```python
from build123d import *

# Parameters (mm, degrees)
BOSS_EXTRU_1_DEPTH             = 15
ESQUISSE3_R                    = 4
BOSS_EXTRU_2_DEPTH             = 20
ESQUISSE4_R                    = 4
BOSS_EXTRU_3_DEPTH             = 20
TROU_TARAUD_M5X0_85_AT_2_COUNT = 2
TROU_TARAUD_M5X0_85_AT_2_PITCH = 44.72135955
ENL_V_START                    = -19
ESQUISSE13_R                   = 4
ESQUISSE13_R_2                 = 3
ENL_V_MAT_EXTRU_1_DEPTH        = 19


with BuildPart() as part:
    # Esquisse1 → Boss.-Extru.1 (new, symmetric)
    with BuildSketch(Plane.XY):
        Polygon((0, 60), (30, 60), (30, 30), (60, 30), (60, 0), (0, 0), align=None)
    extrude(amount=BOSS_EXTRU_1_DEPTH, both=True)

    # Esquisse3 → Boss.-Extru.2 (add)
    with BuildSketch(Plane(origin=(0, 60, 0), x_dir=(-1, 0, 0), z_dir=(0, 1, 0))):
        with Locations(Location((-15, 0, 0), (0, 0, 270))):
            Circle(ESQUISSE3_R)
    extrude(amount=BOSS_EXTRU_2_DEPTH)

    # Esquisse4 → Boss.-Extru.3 (add)
    with BuildSketch(Plane(origin=(60, 0, 0), x_dir=(0, 0, -1), z_dir=(1, 0, 0))):
        with Locations(Location((0, 15, 0), (0, 0, 180))):
            Circle(ESQUISSE4_R)
    extrude(amount=BOSS_EXTRU_3_DEPTH)

    # Esquisse8 → Trou taraudé M5x0.82 (revolve, cut)
    with BuildSketch(Plane(origin=(45, 5, 15), x_dir=(0, -1, 0), z_dir=(1, 0, 0))):
        Polygon((0, 0), (0, 8.2618073), (2.1, 7), (2.1, 0), align=None)
    trou_taraud_m5x0_82 = revolve(axis=Axis((45, 5, 21.35), (0, 0, -1)), mode=Mode.SUBTRACT)

    # Esquisse9 → Trou taraudé M5x0.83 (revolve, cut)
    with BuildSketch(Plane(origin=(45, 25, 15), x_dir=(0, -1, 0), z_dir=(1, 0, 0))):
        Polygon((0, 0), (0, 8.2618073), (2.1, 7), (2.1, 0), align=None)
    trou_taraud_m5x0_83 = revolve(axis=Axis((45, 25, 21.35), (0, 0, -1)), mode=Mode.SUBTRACT)

    # Esquisse10 → Trou taraudé M5x0.84 (revolve, cut)
    with BuildSketch(Plane(origin=(5, 45, 15), x_dir=(0, -1, 0), z_dir=(1, 0, 0))):
        Polygon((0, 0), (0, 8.2618073), (2.1, 7), (2.1, 0), align=None)
    trou_taraud_m5x0_84 = revolve(axis=Axis((5, 45, 21.35), (0, 0, -1)), mode=Mode.SUBTRACT)

    # Esquisse12 → Trou taraudé M5x0.85 (revolve, cut)
    with BuildSketch(Plane(origin=(25, 45, 15), x_dir=(0, -1, 0), z_dir=(1, 0, 0))):
        Polygon((0, 0), (0, 8.2618073), (2.1, 7), (2.1, 0), align=None)
    trou_taraud_m5x0_85 = revolve(axis=Axis((25, 45, 21.35), (0, 0, -1)), mode=Mode.SUBTRACT)

    # Trou taraudé M5x0.85 at 2: Trou taraudé M5x0.85 ×2
    with Locations(*[Vector(-0.447213595499958, -0.8944271909999159, 0) * (i * TROU_TARAUD_M5X0_85_AT_2_PITCH) for i in range(1, TROU_TARAUD_M5X0_85_AT_2_COUNT)]):
        add(trou_taraud_m5x0_85, mode=Mode.SUBTRACT)

    # Symétrie1: Trou taraudé M5x0.82, Trou taraudé M5x0.83, Trou taraudé M5x0.84, Trou taraudé M5x0.85 across plane
    add(trou_taraud_m5x0_82.mirror(Plane.XY), mode=Mode.SUBTRACT)
    add(trou_taraud_m5x0_83.mirror(Plane.XY), mode=Mode.SUBTRACT)
    add(trou_taraud_m5x0_84.mirror(Plane.XY), mode=Mode.SUBTRACT)
    add(trou_taraud_m5x0_85.mirror(Plane.XY), mode=Mode.SUBTRACT)

    # Symétrie1 copy 1 sketch → Symétrie1 copy 1 (revolve, cut)
    with BuildSketch(Plane(origin=(5, 5, -15), x_dir=(0, -1, 0), z_dir=(1, 0, 0))):
        Polygon((0, 0), (0, -8.2618073), (2.1, -7), (2.1, 0), align=None)
    revolve(axis=Axis((5, 5, -21.35), (0, 0, -1)), mode=Mode.SUBTRACT)

    # Esquisse13 → Enlèv. mat.-Extru.1 (cut)
    with BuildSketch(Plane(origin=(80, 0, 0), x_dir=(0, 0, -1), z_dir=(1, 0, 0)).offset(ENL_V_START)):
        with Locations(Location((0, 15, 0), (0, 0, 180))):
            Circle(ESQUISSE13_R)
        with Locations((0, 15)):
            Circle(ESQUISSE13_R_2, mode=Mode.SUBTRACT)
    extrude(amount=ENL_V_MAT_EXTRU_1_DEPTH, mode=Mode.SUBTRACT)


solid = part.part
```
Read the model definition and answer for the solid it produces. Units are mm, in the model's axes. A direction names the side the tool comes from. Coordinates: 2 decimals unless noted, no trailing zeros. Order: outer loops, then holes, each group sorted by start corner. A loop starts at its lowest first (then second) coordinate and runs counter-clockwise, first axis right, second up. Notation, with made-up numbers: (48.25, 74.5) - (92.25, 74.5) arc R32 ccw to (92.25, 109.5) - close; hole circle Ø3 at (-11.75, 4.25). An arc over 180 degrees is marked (long way). Answer as a JSON object with one key per item and string values. Group by question number.
Item 1: Section D-D (x = 71.5) is taken. Give the vertices of the cut face in (y, z).
Item 2: Section B-B (y = 17) is taken. Give the vertices of the cut face in (x, z), plus the area to 3 significant figures.
Item 3: The mould has two halves that part along Y. Classify faces 5 (the face through (44.75, 25.27, -6.96)), 6 (the face through (24, 24, -15)), 7 (the face through (15, 80, 0)): +Y half, -Y half, draft (parallel to the pull), parting line (faces both ways), or undercut.
Item 4: Section C-C (z = -5) is taken. Give the vertices of the cut face in (x, y), plus the area to 3 significant figures.
Item 5: Section A-A (z = 11) is taken. Give the vertices of the cut face in (x, y), plus the area to 3 significant figures.
Item 6: A tool of negligible diameter and unlimited length cuts with its end or side. For faces 1 (the face through (5.8, 43.06, -11.55)), 2 (the face through (30, 45, 0)), 3 (the face through (2.918, 5.273, 11.549)), 4 (the face through (60, 19, 4)), from which of +Z, -Z, +X, -X, +Y, -Y can it reach the whole face along a straight path? Write none if from no direction.
Item 7: Flat-ended cylindrical pins translate along their axes: P1, Ø4, axis at x = 5, y = 45, coming from the +Z side; P2, Ø3.5, axis at x = 25, y = 45, coming from the -Z side; P3, Ø15, axis at x = 46.5, z = -2, coming from the +Y side; P4, Ø12, axis at x = 69, z = -9.5, coming from the +Y side. Find the tip coordinate at first contact, or state that the pin passes through.
Item 8: Consider probe 1 along Y at (x, z) = (5, 12); probe 2 along X at (y, z) = (45, -10.5); probe 3 along Y at (x, z) = (32, 2.75). Determine where each line is inside the solid, lowest interval first. Write a range as from..to.
Results are:
{
 "1": {"outline": "circle Ø6 at (15, 0)"},
 "2": {"outline": "(0, -15) - (60, -15) - (60, -3.46) - (61, -3.46) - (61, -2.24) - (80, -2.24) - (80, 2.24) - (61, 2.24) - (61, 3.46) - (60, 3.46) - (60, 15) - (0, 15) - close", "area": "1,890 mm^2"},
 "3": {"face 5": "undercut", "face 6": "draft", "face 7": "+Y half"},
 "4": {"outline": "(0, 0) - (60, 0) - (60, 30) - (30, 30) - (30, 60) - (0, 60) - close", "area": "2,700 mm^2"},
 "5": {"outline": "(0, 0) - (60, 0) - (60, 30) - (30, 30) - (30, 60) - (0, 60) - close; hole circle Ø4.2 at (5, 5); hole circle Ø4.2 at (5, 45); hole circle Ø4.2 at (25, 45); hole circle Ø4.2 at (45, 5); hole circle Ø4.2 at (45, 25)", "area": "2,630 mm^2"},
 "6": {"face 1": "-Z", "face 2": "+Z, -Z, +X, +Y", "face 3": "+Z", "face 4": "+X"},
 "7": {"P1": "stops at z = 7.94", "P2": "stops at z = -7.79", "P3": "stops at y = 30", "P4": "passes through"},
 "8": {"probe 1": "y = 0..2.9, 7.1..42.9, 47.1..60", "probe 2": "x = 0..2.9, 7.1..22.9, 27.1..30", "probe 3": "y = 0..30"}
}
